Source: CAD feature listing. Evaluate the final solid. Frame: model axes, mm. Face numbers are marked on the shaded views. A direction names the side the tool comes from. Give positions to 0.01 mm unless a question says otherwise; leave off trailing zeros. Order: outer loops, then holes, each group sorted by start corner. A loop starts at its lowest first (then second) coordinate and runs counter-clockwise, first axis right, second up. Notation, with made-up numbers: (79, -33.75) -> (113, -33.75) arc R30 ccw to (113, -10.75) -> close; hole circle Ø10 at (-7, 74.25). An arc over 180 degrees is marked (long way). Use CSV: the item, a comma, the result in double quotes.
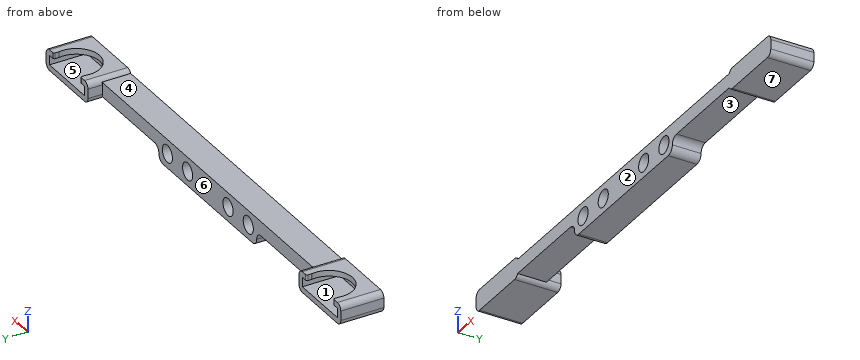
```python
from build123d import *

# Parameters (mm, degrees)
SKIZZE1_W                                   = 29
SKIZZE1_H                                   = 10
SKIZZE1_R                                   = 3
AUFSATZ_LINEAR_AUSTRAGEN1_DEPTH             = 10
SKIZZE2_W                                   = 5
SKIZZE2_H                                   = 10
AUFSATZ_LINEAR_AUSTRAGEN2_DEPTH             = 57.25
SKIZZE3_W                                   = 20.8
SKIZZE3_H                                   = 3.3
SCHNITT_LINEAR_AUSTRAGEN1_DEPTH             = 8
AUFSATZ_LINEAR_AUSTRAGEN3_REACH             = 88.972
SKIZZE5_W                                   = 24.8
SKIZZE5_H                                   = 7.3
SKIZZE5_W_2                                 = 20.8
SKIZZE5_H_2                                 = 3.3
AUFSATZ_LINEAR_AUSTRAGEN3_DIRECTION_2_DEPTH = 5
SCHNITT_LINEAR_AUSTRAGEN2_REACH             = 91.376
SKIZZE4_R                                   = 8.075
SCHNITT_LINEAR_START                        = -1.834682
SKIZZE7_W                                   = 15.9
SKIZZE7_H                                   = 2
SCHNITT_LINEAR_AUSTRAGEN3_DEPTH             = 1.834682
VERRUNDUNG1_R                               = 2
VERRUNDUNG3_R                               = 0.5
VERRUNDUNG1_OF_SPIEGELN1_R                  = 2
VERRUNDUNG3_OF_SPIEGELN1_R                  = 0.5
VERRUNDUNG2_START                           = -1
VERRUNDUNG2_DEPTH                           = 12
VERRUNDUNG2_2_DEPTH                         = 10


with BuildPart() as part:
    # Skizze1 → Aufsatz-Linear austragen1 (new body)
    # profile 1 of 2: a face of its own
    with BuildSketch(Plane(origin=(0, 0, 0), x_dir=(1, 0, 0), z_dir=(0, 1, 0))):
        with Locations((-14.5, 0)):
            Rectangle(SKIZZE1_W, SKIZZE1_H)
        with Locations(Location((-24, 0, 0), (0, 0, 270))):
            Circle(SKIZZE1_R, mode=Mode.SUBTRACT)
        with Locations(Location((-12, 0, 0), (0, 0, 270))):
            Circle(SKIZZE1_R, mode=Mode.SUBTRACT)
    # profile 2 of 2: a face of its own
    with BuildSketch(Plane(origin=(0, 0, 0), x_dir=(1, 0, 0), z_dir=(0, 1, 0))):
        with Locations((14.5, 0)):
            Rectangle(SKIZZE1_W, SKIZZE1_H)
        with Locations(Location((12, 0, 0), (0, 0, 270))):
            Circle(SKIZZE1_R, mode=Mode.SUBTRACT)
        with Locations(Location((24, 0, 0), (0, 0, 270))):
            Circle(SKIZZE1_R, mode=Mode.SUBTRACT)
    extrude(amount=AUFSATZ_LINEAR_AUSTRAGEN1_DEPTH)

    # Skizze2 → Aufsatz-Linear austragen2 (add)
    with BuildSketch(Plane(origin=(29, 0, 0), x_dir=(0, 0, -1), z_dir=(1, 0, 0))):
        with Locations((-2.5, 5)):
            Rectangle(SKIZZE2_W, SKIZZE2_H)
    aufsatz_linear_austragen2 = extrude(amount=AUFSATZ_LINEAR_AUSTRAGEN2_DEPTH)

    # Skizze3 → Schnitt-Linear austragen1 (cut)
    with BuildSketch(Plane(origin=(0, 10, 0), x_dir=(1, 0, 0), z_dir=(0, 1, 0))):
        with Locations((75, -2.5)):
            Rectangle(SKIZZE3_W, SKIZZE3_H)
    schnitt_linear_austragen1 = extrude(amount=-SCHNITT_LINEAR_AUSTRAGEN1_DEPTH, mode=Mode.SUBTRACT)

    # Aufsatz-Linear austragen3: up to this face of the body (flat: up to its plane)
    aufsatz_linear_austragen3_end = Plane(part.part.faces().sort_by_distance((28.625, 0, 3.84316974))[0])
    # Skizze5 → Aufsatz-Linear austragen3 (add, up to the picked face)
    with BuildSketch(Plane(origin=(0, 10, 0), x_dir=(1, 0, 0), z_dir=(0, 1, 0)), mode=Mode.PRIVATE) as aufsatz_linear_austragen3_sk1:
        with Locations((75, -2.5)):
            Rectangle(SKIZZE5_W, SKIZZE5_H)
        with Locations((75, -2.5)):
            Rectangle(SKIZZE5_W_2, SKIZZE5_H_2, mode=Mode.SUBTRACT)
    aufsatz_linear_austragen3_tool1 = split(extrude(aufsatz_linear_austragen3_sk1.sketch, amount=-AUFSATZ_LINEAR_AUSTRAGEN3_REACH, mode=Mode.PRIVATE), bisect_by=aufsatz_linear_austragen3_end, keep=Keep.BOTH, mode=Mode.PRIVATE)
    aufsatz_linear_austragen3 = aufsatz_linear_austragen3_tool1.solids().sort_by(Axis((75, 10, 5.891479), (0, -1, 0)))[0]
    add(aufsatz_linear_austragen3)

    # Skizze5 → Aufsatz-Linear austragen3 direction 2 (add)
    with BuildSketch(Plane(origin=(0, 10, 0), x_dir=(1, 0, 0), z_dir=(0, 1, 0))):
        with Locations((75, -2.5)):
            Rectangle(SKIZZE5_W, SKIZZE5_H)
        with Locations((75, -2.5)):
            Rectangle(SKIZZE5_W_2, SKIZZE5_H_2, mode=Mode.SUBTRACT)
    aufsatz_linear_austragen3_direction_2 = extrude(amount=AUFSATZ_LINEAR_AUSTRAGEN3_DIRECTION_2_DEPTH)

    # Skizze4 → Schnitt-Linear austragen2 (cut, up to next)
    with BuildSketch(Plane.XY.offset(6.15), mode=Mode.PRIVATE) as schnitt_linear_austragen2_sk1:
        with Locations((75, 11.75)):
            Circle(SKIZZE4_R)
    schnitt_linear_austragen2_tool1 = extrude(schnitt_linear_austragen2_sk1.sketch, amount=-SCHNITT_LINEAR_AUSTRAGEN2_REACH, mode=Mode.PRIVATE) & part.part
    schnitt_linear_austragen2 = schnitt_linear_austragen2_tool1.solids().sort_by_distance((75, 11.75, 6.15))[0]
    add(schnitt_linear_austragen2, mode=Mode.SUBTRACT)

    # Skizze7 → Schnitt-Linear austragen3 (cut)
    with BuildSketch(Plane(origin=(0, 15, 0), x_dir=(1, 0, 0), z_dir=(0, 1, 0)).offset(SCHNITT_LINEAR_START)):
        with Locations((75, -5.15)):
            Rectangle(SKIZZE7_W, SKIZZE7_H)
    schnitt_linear_austragen3 = extrude(amount=SCHNITT_LINEAR_AUSTRAGEN3_DEPTH, mode=Mode.SUBTRACT)

    # Verrundung1
    verrundung1_edges = [part.edges().sort_by_distance(p)[0] for p in [
        (87.4, 7.5, 6.15),
        (87.4, 7.5, -1.15),
        (62.6, 7.5, 6.15),
        (62.6, 7.5, -1.15),
    ]]
    fillet(verrundung1_edges, radius=VERRUNDUNG1_R)

    # Verrundung3
    verrundung3_edges = [part.edges().sort_by_distance(p)[0] for p in [
        (82.95, 15, 5.15),
        (82.95, 13.165318, 5.15),
        (67.05, 15, 5.15),
        (67.05, 13.165318, 5.15),
    ]]
    fillet(verrundung3_edges, radius=VERRUNDUNG3_R)

    # Spiegeln1: Aufsatz-Linear austragen2, Schnitt-Linear austragen1, Aufsatz-Linear austragen3, Aufsatz-Linear austragen3 direction 2, Schnitt-Linear austragen2, Schnitt-Linear austragen3 across plane
    add(aufsatz_linear_austragen2.mirror(Plane(origin=(0, 0, 0), x_dir=(0, 0, 1), z_dir=(1, 0, 0))))
    add(schnitt_linear_austragen1.mirror(Plane(origin=(0, 0, 0), x_dir=(0, 0, 1), z_dir=(1, 0, 0))), mode=Mode.SUBTRACT)
    add(aufsatz_linear_austragen3.mirror(Plane(origin=(0, 0, 0), x_dir=(0, 0, 1), z_dir=(1, 0, 0))))
    add(aufsatz_linear_austragen3_direction_2.mirror(Plane(origin=(0, 0, 0), x_dir=(0, 0, 1), z_dir=(1, 0, 0))))
    add(schnitt_linear_austragen2.mirror(Plane(origin=(0, 0, 0), x_dir=(0, 0, 1), z_dir=(1, 0, 0))), mode=Mode.SUBTRACT)
    add(schnitt_linear_austragen3.mirror(Plane(origin=(0, 0, 0), x_dir=(0, 0, 1), z_dir=(1, 0, 0))), mode=Mode.SUBTRACT)

    # Verrundung1 of Spiegeln1
    verrundung1_of_spiegeln1_edges = [part.edges().sort_by_distance(p)[0] for p in [
        (-87.4, 7.5, 6.15),
        (-87.4, 7.5, -1.15),
        (-62.6, 7.5, 6.15),
        (-62.6, 7.5, -1.15),
    ]]
    fillet(verrundung1_of_spiegeln1_edges, radius=VERRUNDUNG1_OF_SPIEGELN1_R)

    # Verrundung3 of Spiegeln1
    verrundung3_of_spiegeln1_edges = [part.edges().sort_by_distance(p)[0] for p in [
        (-82.95, 15, 5.15),
        (-82.95, 13.165318, 5.15),
        (-67.05, 15, 5.15),
        (-67.05, 13.165318, 5.15),
    ]]
    fillet(verrundung3_of_spiegeln1_edges, radius=VERRUNDUNG3_OF_SPIEGELN1_R)

    # Verrundung2: read off the stored shape, not the designer's step
    # Verrundung2 outline → Verrundung2 (cut)
    with BuildSketch(Plane(origin=(0, 0, 0), x_dir=(1, 0, 0), z_dir=(0, 1, 0)).offset(VERRUNDUNG2_START)):
        with BuildLine():
            ThreePointArc((-29, 2.5), (-28.267766953, 4.267766953), (-26.5, 5))
            Line((-26.5, 5), (-29, 5))
            Line((-29, 5), (-29, 2.5))
        make_face()
        with BuildLine():
            ThreePointArc((26.5, 5), (28.267766953, 4.267766953), (29, 2.5))
            Line((29, 2.5), (29, 5))
            Line((29, 5), (26.5, 5))
        make_face()
    extrude(amount=VERRUNDUNG2_DEPTH, mode=Mode.SUBTRACT)

    # Verrundung2 2 outline → Verrundung2 2 (add)
    with BuildSketch(Plane(origin=(0, 0, 0), x_dir=(1, 0, 0), z_dir=(0, 1, 0))):
        with BuildLine():
            Line((-29, 0), (-29, 2.5))
            ThreePointArc((-29, 2.5), (-29.732233047, 0.732233047), (-31.5, 0))
            Line((-31.5, 0), (-29, 0))
        make_face()
        with BuildLine():
            ThreePointArc((31.5, 0), (29.732233047, 0.732233047), (29, 2.5))
            Line((29, 2.5), (29, 0))
            Line((29, 0), (31.5, 0))
        make_face()
    extrude(amount=VERRUNDUNG2_2_DEPTH)


solid = part.part
```
1. Access query for the marked faces 4, 5, 6 and 7. Directions: +Z, -Z, +X, -X, +Y, -Y. A direction counts if a zero-diameter tool reaches every point of the face in a straight line with its end or side. Return the directions, or none.
Answer below:
face 4,"+Z, +Y, -Y"
face 5,"+Y"
face 6,"+Z, -Z, +Y"
face 7,"-Z, +X, +Y, -Y"
2. Section query A-A on x = -24. Return loops of the section in (y, z), plus the area to 3 significant figures.
Answer below:
outline,"(0, -5) -> (10, -5) -> (10, -3) -> (0, -3) -> close; (0, 3) -> (10, 3) -> (10, 5) -> (0, 5) -> close"
area,"40.0 mm²"
3. Ray query, line 1 along X through (y, z) = (11.25, 3); line 2 along Z through (x, y) = (73, 12.5); line 3 along Y through (x, z) = (-53, 3.75). Return the intervals inside material, ascending.
Answer below:
line 1,"x = -87.4 to -85.4, -64.6 to -62.6, 62.6 to 64.6, 85.4 to 87.4"
line 2,"z = -1.15 to 0.85"
line 3,"y = 0 to 10"
4. Section query B-B on x = -75. Return loops of the section in (y, z) (3 decimals), plus the area to 4 significant figures.
Answer below:
outline,"(0, -1.15) -> (15, -1.15) -> (15, 0.85) -> (2, 0.85) -> (2, 4.15) -> (3.675, 4.15) -> (3.675, 6.15) -> (0, 6.15) -> close"
area,"43.95 mm²"
5. Section query C-C on x = 3. Return loops of the section in (y, z).
Answer below:
outline,"(0, -5) -> (10, -5) -> (10, 5) -> (0, 5) -> close"
6. Section query D-D on x = -52. Return loops of the section in (y, z).
Answer below:
outline,"(0, 0) -> (10, 0) -> (10, 5) -> (0, 5) -> close"
7. Mould query, pull axis X, two halves, no side actions, for the marked faces 1, 2 and 3. Classes: released by +X, released by -X, zero draft, split by the parting line, or undercut.
Answer below:
face 1,"undercut"
face 2,"zero draft"
face 3,"undercut"
8. Pin query (flat end, axial travel): P1, Ø4, axis at x = 75.5, y = 7, coming from the +Z side; P2, Ø2, axis at y = 2.5, z = -1.5, coming from the +X side; P3, Ø5, axis at x = -24, z = 0, coming from the +Y side; P4, Ø1, axis at y = 14, z = 5, coming from the -X side. Return the tip coordinate at first contact, or that it passes through.
Answer below:
P1,"stops at z = 0.85"
P2,"stops at x = 86.88"
P3,"passes through"
P4,"stops at x = -87.37"
